```python
from build123d import *

# Parameters (mm, degrees)
BOSS_EXTRUDE1_START = 15
BOSS_EXTRUDE1_DEPTH = 15
CIRPATTERN1_COUNT   = 8
SKETCH4_R           = 3
BOSS_EXTRUDE2_DEPTH = 15
SKETCH5_R           = 1.58775
CUT_EXTRUDE1_DEPTH  = 11.4
FILLET3_R           = 2


with BuildPart() as part:
    # Sketch1 → Revolve1 (revolve)
    with BuildSketch(Plane(origin=(0, 0, 0), x_dir=(1, 0, 0), z_dir=(0, 1, 0)), mode=Mode.PRIVATE) as revolve1_sk:
        with BuildLine():
            Line((0, 0), (0, 30))
            Line((0, 30), (-3, 30))
            Line((-3, 30), (-3, 5))
            Line((-3, 5), (-8, 5))
            ThreePointArc((-8, 5), (-10.828427125, 3.828427125), (-12, 1))
            Line((-12, 1), (-12, 0))
            Line((-12, 0), (0, 0))
        make_face()
    revolve(revolve1_sk.sketch.rotate(Axis((-12, 0, 0), (1, 0, 0)), 180), axis=Axis((-12, 0, 0), (1, 0, 0)))

    # Sketch2 → Boss-Extrude1 (add)
    with BuildSketch(Plane.ZY.offset(3).offset(BOSS_EXTRUDE1_START)):
        with BuildLine():
            ThreePointArc((-6.74081952, 9.317260982), (-7.459861891, 8.752168906), (-8.131727984, 8.131727984))
            ThreePointArc((-8.131727984, 8.131727984), (-8.088596883, 20.561719247), (0, 30))
            ThreePointArc((0, 30), (1.848623078, 29.942989041), (3.690220038, 29.772172848))
            ThreePointArc((3.690220038, 29.772172848), (-5.738161973, 21.693077802), (-6.74081952, 9.317260982))
        make_face()
    boss_extrude1 = extrude(amount=-BOSS_EXTRUDE1_DEPTH)

    # CirPattern1: Boss-Extrude1 ×8 about axis
    cirpattern1_axis = Axis((0, 0, 0), (1, 0, 0))
    for i in range(1, CIRPATTERN1_COUNT):
        add(boss_extrude1.rotate(cirpattern1_axis, i * 360 / CIRPATTERN1_COUNT))

    # Sketch4 → Boss-Extrude2 (add)
    with BuildSketch(Plane(origin=(0, 0, 0), x_dir=(0, 0, -1), z_dir=(1, 0, 0))):
        with Locations(Location((0, 0, 0), (0, 0, 180))):
            Circle(SKETCH4_R)
    extrude(amount=BOSS_EXTRUDE2_DEPTH)

    # Sketch5 → Cut-Extrude1 (cut)
    with BuildSketch(Plane(origin=(15, 0, 0), x_dir=(0, 0, -1), z_dir=(1, 0, 0))):
        Circle(SKETCH5_R)
    extrude(amount=-CUT_EXTRUDE1_DEPTH, mode=Mode.SUBTRACT)

    # Fillet3
    fillet3_edges = [part.edges().sort_by_distance(p)[0] for p in [
        (0, 0, -3),
    ]]
    fillet(fillet3_edges, radius=FILLET3_R)


solid = part.part
```
Part model, mm, in its own coordinate system. A direction names the side the tool comes from. Coordinates: 2 decimals unless noted, no trailing zeros. Order: outer loops, then holes, each group sorted by start corner. A loop starts at its lowest first (then second) coordinate and runs counter-clockwise, first axis right, second up. Notation, with made-up numbers: (72.25, 86.25) - (104.25, 86.25) arc R21 ccw to (104.25, 110.25) - close; hole circle Ø7 at (37, 26). An arc over 180 degrees is marked (long way). Return JSON: item names as keys, results as strings. Group by question number.
Item 1: Pin check, flat tips, straight feed: pin 1 (3 mm diameter, centred on y = 0, z = 0, fed in from -X); pin 2 (4 mm diameter, centred on x = 4.5, y = 0, fed in from +Z); pin 3 (12 mm diameter, centred on x = -10.5, z = 11.5, fed in from -Y); pin 4 (2 mm diameter, centred on x = 1.5, y = 23.5, fed in from +Z). Stop position of each tip, or through.
Item 2: Cut at A-A (x = -15). State how many separate pieces and enclosed holes the cut face has, plus the area to 3 significant figures.
Item 3: Cut at C-C (z = -17.5). List the corners of the cut face in (x, y), plus the area to 3 significant figures.
Item 4: Cut at D-D (x = 11.5). List the corners of the cut face in (y, z), plus the area to 3 significant figures.
Item 5: Pull direction Y, two halves, no side cores. Call faces 1 (the face through (8.41, -0.9, 2.86)), 2 (the face through (-10.6, 11.45, -19.45)), 3 (the face through (-18, -7, -22)): pulls with the +Y half, pulls with the -Y half, needs draft (parallel to the pull), parting line crosses it, or undercut.
Item 6: Which spindle directions (+Z, -Z, +X, -X, +Y, -Y) get a long thin tool onto all of the face, cutting with end or side? Do faces 4 (the face through (-18, -22, 7)), 5 (the face through (-10.605, -11.463, -0.927)). Say none if no direction does.
Item 7: Drill centre lines: probe 1 along Z at (x, y) = (-13.5, 12); probe 2 along Y at (x, z) = (7, 0); probe 3 along X at (y, z) = (-18.5, 14.5). Where is each one in solid material? Low to high. Write a range as from..to.
Check values:
{
 "1": {"pin 1": "stops at x = -12", "pin 2": "stops at z = 3", "pin 3": "stops at y = -25.24", "pin 4": "passes through"},
 "2": {"separate pieces": "8", "enclosed holes": "0", "area": "345 mm2"},
 "3": {"outline": "(-18, -21.85) - (-3, -21.85) - (-3, -24.37) - (0, -24.37) - (0, 24.37) - (-3, 24.37) - (-3, 7.34) - (-18, 7.34) - (-18, 4.53) - (-3, 4.53) - (-3, -7.2) - (-18, -7.2) - (-18, -8.93) - (-3, -8.93) - (-3, -20.15) - (-18, -20.15) - close", "area": "240 mm2"},
 "4": {"outline": "circle Ø6 at (0, 0); hole circle Ø3.18 at (0, 0)", "area": "20.4 mm2"},
 "5": {"face 1": "parting line crosses it", "face 2": "undercut", "face 3": "needs draft"},
 "6": {"face 4": "+Z, -Z, -X, +Y, -Y", "face 5": "-X"},
 "7": {"probe 1": "z = -21.37..-19.61, -9.07..-7.36, 0.24..2.17", "probe 2": "y = -3..-1.59, 1.59..3", "probe 3": "x = -3..0"}
}
